Autodesk Inventor part; units mm, degrees
ref_plane "YZ Plane" through (0, 0, 0) normal (1, 0, 0) x (0, 1, 0)
ref_plane "XZ Plane" through (0, 0, 0) normal (0, 1, 0) x (-1, 0, 0)
ref_plane "XY Plane" through (0, 0, 0) normal (0, 0, 1) x (1, 0, 0)
sketch "Sketch1" plane through (0, 0, 0) normal (0, 0, 1) x (1, 0, 0)
  circle A0 centre (0, 0) radius 1.425
  circle A1 centre (30, 0) radius 1.425
  line L0 (0, 0) -> (30, 0) construction
  line L1 (15, 0) -> (15, -17.6441)
  line L2 (-2.85, 2.85) -> (32.85, 2.85)
  line L3 (32.85, 2.85) -> (32.85, -26.4898)
  line L4 (-2.85, -26.4898) -> (-2.85, 2.85)
  line L5 (2.85, -26.4898) -> (2.85, -3.8397)
  line L6 (2.85, -3.8397) -> (6.5383, 0)
  line L7 (6.5383, 0) -> (23.4617, 0)
  line L8 (23.4617, 0) -> (27.15, -3.8397)
  line L9 (27.15, -3.8397) -> (27.15, -26.4898)
  line L10 (32.85, -26.4898) -> (27.15, -26.4898)
  line L11 (2.85, -26.4898) -> (-2.85, -26.4898)
  dimension "d0" = 2.85
  dimension "d1" = 30
  dimension "d2" = 2.85
  dimension "d3" = 2.85
  dimension "d4" = 2.85
extrude "Extrusion1" add sketch "Sketch1" along normal blind 3
fillet "Fillet1" radius 1 10 edges at (-2.85, 2.85, 1.5) (32.85, 2.85, 1.5) (-2.85, -26.4898, 1.5) (2.85, -26.4898, 1.5) (32.85, -26.4898, 1.5) (27.15, -26.4898, 1.5) (2.85, -3.8397, 1.5) (6.5383, 0, 1.5) (23.4617, 0, 1.5) (27.15, -3.8397, 1.5)
properties part number "ExtraBoardSpacer"
Check sheet for the modelled part. Datum: model origin and axes. Units: mm. A direction names the side the tool comes from. Round coordinates to 2 decimals unless told otherwise and drop trailing zeros. Write each loop counter-clockwise with the first axis right and the second up, starting at its lowest first coordinate (ties: lowest second). Pieces come first, ordered by that corner, then holes. Notation, with made-up numbers: (48, -20) - (63, -20) arc R16 ccw to (63, 8) - close; hole circle Ø4 at (31, 69.25). An arc over 180 degrees is marked (long way). Return JSON: item names as keys, results as strings.
Q1. Cross-section at A-A (x = 30). Record the boundary of the cut face in (y, z) (3 decimals).
Returned:
{"outline": "(-26.49, 0) - (-1.425, 0) - (-1.425, 3) - (-26.49, 3) - close; (1.425, 0) - (2.85, 0) - (2.85, 3) - (1.425, 3) - close"}
Q2. Cross-section at C-C (z = 0.95). Record the boundary of the cut face in (x, y) (3 decimals).
Returned:
{"outline": "(-2.85, -25.49) arc R1 ccw to (-1.85, -26.49) - (1.85, -26.49) arc R1 ccw to (2.85, -25.49) - (2.85, -4.242) arc R1 cw to (3.129, -3.549) - (6.243, -0.307) arc R1 cw to (6.964, 0) - (23.036, 0) arc R1 cw to (23.757, -0.307) - (26.871, -3.549) arc R1 cw to (27.15, -4.242) - (27.15, -25.49) arc R1 ccw to (28.15, -26.49) - (31.85, -26.49) arc R1 ccw to (32.85, -25.49) - (32.85, 1.85) arc R1 ccw to (31.85, 2.85) - (-1.85, 2.85) arc R1 ccw to (-2.85, 1.85) - close; hole circle Ø2.85 at (0, 0); hole circle Ø2.85 at (30, 0)"}
Q3. Access from +Z, -Z, +X, -X, +Y, -Y to the whole of each face (thin tool, end or side, straight path). Record for faces 5 (the flat face through (0, -26.49, 1)), 6 (the flat face through (27.15, -15, 1)).
Returned:
{"face 5": "+Z, -Z, +X, -X, -Y", "face 6": "+Z, -Z, -Y"}
Q4. Cross-section at D-D (x = 8). Record the boundary of the cut face in (y, z).
Returned:
{"outline": "(0, 0) - (2.85, 0) - (2.85, 3) - (0, 3) - close"}
Q5. Draft check along X on faces 1 (the flat face through (4.664, -1.951, 1.479)), 2 (the cylindrical face through (27.435, -26.189, 1.521)), 3 (the flat face through (14, 1, 3)), 4 (the cylindrical face through (-2.565, -26.189, 1.521)). Enter one of: released by +X, released by -X, zero draft, split by the parting line, or undercut.
Returned:
{"face 1": "undercut", "face 2": "undercut", "face 3": "zero draft", "face 4": "released by -X"}
Q6. Scan lines: L1, parallel to X at y = -22.75, z = 0.3; L2, parallel to Y at x = 0, z = 1.5 (3 decimals); L3, parallel to X at y = -0.5, z = 0.55. Record each from-to range of solid material in increasing order. Write a range as from..to.
Returned:
{"L1": "x = -2.85..2.85, 27.15..32.85", "L2": "y = -26.49..-1.425, 1.425..2.85", "L3": "x = -2.85..-1.33, 1.33..6.06, 23.94..28.67, 31.33..32.85"}
Q7. Depth check by flat-ended pin: P1, Ø1.5, axis at x = 18, z = 1.5, coming from the -Y side. Enter the tip coordinate at first touch or a pass-through.
Returned:
{"P1": "stops at y = 0"}
Q8. Cross-section at B-B (y = -11). Record the boundary of the cut face in (x, z).
Returned:
{"outline": "(-2.85, 0) - (2.85, 0) - (2.85, 3) - (-2.85, 3) - close; (27.15, 0) - (32.85, 0) - (32.85, 3) - (27.15, 3) - close"}
